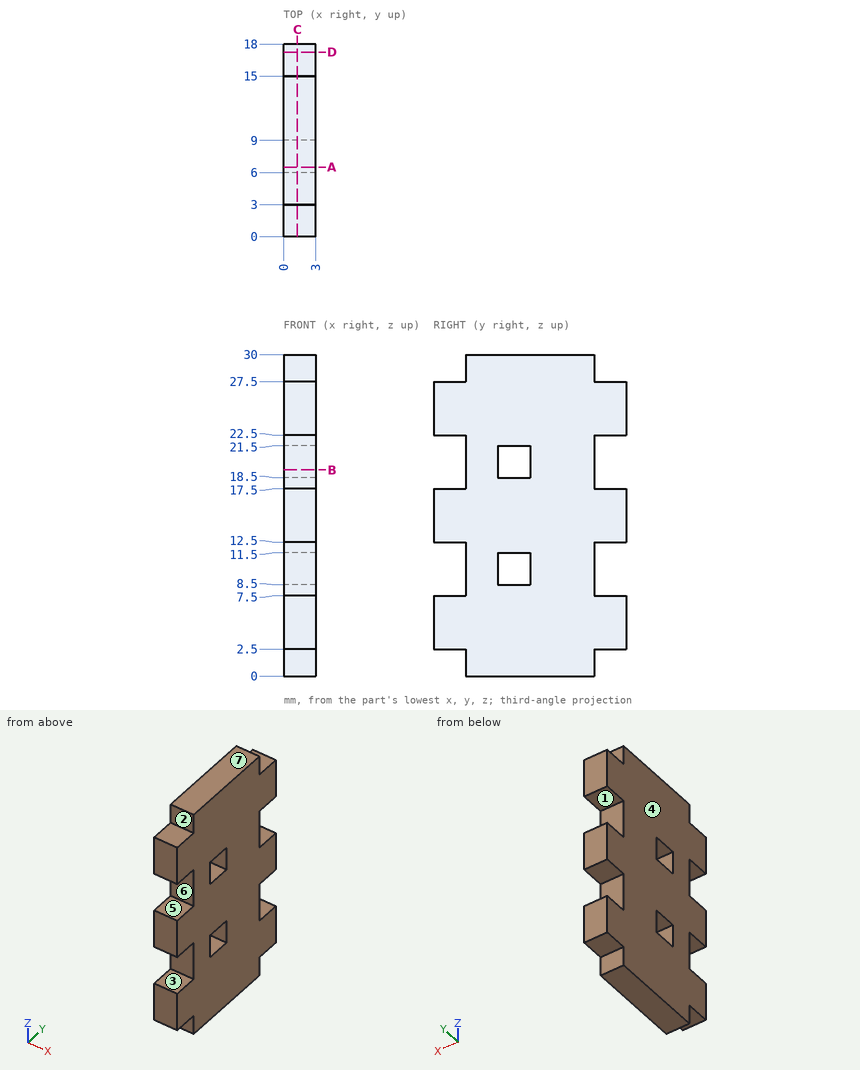
Could you check a few things on this drawing? It's one solid part, dimensions in mm from its lowest x, y, z. A direction names the side the tool comes from. Give positions to 0.01 mm unless a question says otherwise; leave off trailing zeros. Order: outer loops, then holes, each group sorted by start corner. A loop starts at its lowest first (then second) coordinate and runs counter-clockwise, first axis right, second up. Notation, with made-up numbers: M 31,-38 L 87,-38 A33 ccw 87,-10 Z; hole C 68,29.5 d11. An arc over 180 degrees is marked long. Use one line per item in the form item = value. Start each with the question number.
Item 1: If we section it at B-B (z = 19.25): Write out the boundary of the cut face in (x, y).
Item 2: Will these pins go through, and if not, where does the flat tip stop? pin 1 Ø1.5 at (x, z) = (1, 19) entering from -Y; pin 2 Ø0.9 at (x, y) = (1, 1.5) entering from -Z; pin 3 Ø1 at (x, z) = (2.5, 19.5) entering from +Y.
Item 3: If we section it at C-C (x = 1.3): State how many separate pieces and enclosed holes the cut face has, then the cut area to 3 significant figures.
Item 4: We'd pull the mould along Z, two halves only. Please class the marked faces 4, 5, 6 and 7: +Z half, -Z half, draft (parallel to the pull), parting line (faces both ways), or undercut.
Item 5: If we section it at A-A (y = 6.5): Write out the boundary of the cut face in (x, z).
Item 6: If I drill on line 1 along Z through (x, y) = (2.8, 16.25); line 2 along Z through (x, y) = (0.35, 6.75); line 3 along Y through (x, z) = (1.1, 8.75), over which ranges is the centre line in solid material (lowest first)?
Item 7: For the marked faces 1, 2 and 3, which set-ups out of +Z, -Z, +X, -X, +Y, -Y let a thin tool reach every point of the face, with its end or its side?
Item 8: If we section it at D-D (y = 17.25): Write out the boundary of the cut face in (x, z).
Outcome:
q1.outline = M 0,3 L 3,3 L 3,6 L 0,6 Z; M 0,9 L 3,9 L 3,15 L 0,15 Z
q2.pin_1 = 3
q2.pin_2 = 2.5
q2.pin_3 = 15
q3.separate_pieces = 1
q3.enclosed_holes = 2
q3.area = 432 mm2
q4.face_4 = draft
q4.face_5 = undercut
q4.face_6 = undercut
q4.face_7 = +Z half
q5.outline = M 0,0 L 3,0 L 3,8.5 L 0,8.5 Z; M 0,11.5 L 3,11.5 L 3,18.5 L 0,18.5 Z; M 0,21.5 L 3,21.5 L 3,30 L 0,30 Z
q6.line_1 = 2.5 to 7.5, 12.5 to 17.5, 22.5 to 27.5
q6.line_2 = 0 to 8.5, 11.5 to 18.5, 21.5 to 30
q6.line_3 = 3 to 6, 9 to 15
q7.face_1 = +X, -X, +Y
q7.face_2 = +Z, +X, -X, -Y
q7.face_3 = +X, -X, -Y
q8.outline = M 0,2.5 L 3,2.5 L 3,7.5 L 0,7.5 Z; M 0,12.5 L 3,12.5 L 3,17.5 L 0,17.5 Z; M 0,22.5 L 3,22.5 L 3,27.5 L 0,27.5 Z
